Autodesk Inventor part; units mm, degrees
ref_plane "YZ Plane" through (0, 0, 0) normal (1, 0, 0) x (0, 1, 0)
ref_plane "XZ Plane" through (0, 0, 0) normal (0, 1, 0) x (-1, 0, 0)
ref_plane "XY Plane" through (0, 0, 0) normal (0, 0, 1) x (1, 0, 0)
sketch "Sketch1" plane through (0, 0, 0) normal (0, 0, 1) x (1, 0, 0)
  circle A0 centre (0, 0) radius 3.5687
  arc A1 (-6.4809, -2.9901) -> (6.4801, -2.9918) centre (0, 0) ccw
  line L0 (-20.3315, 22.225) -> (23.7148, 22.225)
  circle A2 centre (0, 44.45) radius 3.5687
  arc A3 (6.4801, 47.4418) -> (-6.4809, 47.4401) centre (0, 44.45) ccw
  circle A4 centre (0, 22.225) radius 14.8487
  circle A5 centre (0, 22.225) radius 13.5003
  line L1 (-18.1146, 22.225) -> (-6.4809, 47.4401)
  line L2 (18.1226, 22.225) -> (6.4801, 47.4418)
  line L3 (-18.1146, 22.225) -> (-6.4809, -2.9901)
  line L4 (18.1226, 22.225) -> (6.4801, -2.9918)
  point P0 (-14.3353, 14.0338)
  point P1 (14.3408, 14.0338)
  dimension "d0" = 7.1374
  dimension "d1" = 14.2748
  dimension "d2" = 44.45
extrude "Extrusion1" add sketch "Sketch1" against normal blind 1.6002
sketch "Sketch2" plane through (0, 0, 0) normal (1, 0, 0) x (0, 1, 0)
  point P0 (0, 0)
sketch "Sketch3" plane through (0, 0, 0) normal (1, 0, 0) x (0, 1, 0)
  arc A0 (35.7382, 2.1018) -> (35.0472, 13.022) centre (22.225, 6.7287) ccw
  line L0 (51.5874, 0) -> (47.4401, 0)
  line L1 (51.5874, 0) -> (34.4832, 0)
  line L2 (-2.9901, 0) -> (-7.1374, 0)
  line L3 (-7.1374, 0) -> (7.1476, 1.1293)
  line L4 (33.3323, 12.8864) -> (35.0472, 13.022)
  arc A1 (35.7382, 2.1018) -> (37.2401, 0) centre (37.2401, 1.5875) ccw
  line L5 (48.0187, -1.6002) -> (40.8813, -1.6002)
  line L6 (3.5687, -1.6002) -> (-3.5687, -1.6002)
  line L7 (22.225, -1.6002) -> (-2.9901, -1.6002)
  line L8 (47.4401, -1.6002) -> (22.225, -1.6002)
  line L9 (47.4418, -1.6002) -> (47.4401, -1.6002)
  line L10 (22.225, -1.6002) -> (47.4418, -1.6002)
  line L11 (-2.9918, -1.6002) -> (22.225, -1.6002)
  line L12 (-2.9901, -1.6002) -> (-2.9918, -1.6002)
  arc A2 (34.2371, 2.6056) -> (33.3323, 12.8864) centre (22.225, 6.7287) ccw
  line L13 (51.5874, -1.6002) -> (47.4401, -1.6002)
  line L14 (51.5874, -1.6002) -> (37.2401, -1.6002)
  arc A3 (34.2371, 2.6056) -> (34.4832, 0) centre (37.2401, 1.5748) ccw
  line L15 (22.225, -1.6002) -> (22.225, 16.2984)
  arc A4 (34.4832, 0) -> (37.2401, -1.6002) centre (37.2401, 1.5748) ccw
  line L16 (37.2401, -1.6002) -> (22.225, -1.6002)
  line L17 (34.4832, 0) -> (22.225, 0)
  point P0 (0, 0)
  point P1 (47.4418, 0)
  point P2 (-2.9918, 0)
  point P3 (31.8125, -1.6002)
  dimension "d28" = 1.5875
  dimension "d29" = 3.175
revolve "Revolution2" add sketch "Sketch3" angle 360 about axis through (0, 22.225, -1.6002) along (0, 0, 1) contours A1 L1 A3 A2 L4 A0
revolve "Revolution3" cut sketch "Sketch3" angle 360 about axis through (0, 22.225, -1.6002) along (0, 0, 1) contours A4 L8 L15 L17
sketch "Sketch4" plane through (0, 0, 0) normal (0, 0, 1) x (1, 0, 0)
  line L0 (6.4801, -2.9918) -> (18.1226, 22.225)
  line L1 (18.1226, 22.225) -> (6.4801, 47.4418)
  circle A0 centre (0, 44.45) radius 3.5687
  circle A1 centre (0, 22.225) radius 15.0151
  line L2 (0, 44.45) -> (0, 57.4596)
  line L3 (-14.2875, 44.45) -> (-14.2875, 57.4596)
  arc A2 (14.2875, 30.5316) -> (14.2875, 26.8424) centre (18.632, 28.687) ccw
  arc A3 (14.2875, 17.6076) -> (14.2875, 26.8424) centre (0, 22.225) ccw
  arc A4 (14.2875, 17.6076) -> (14.2875, 13.9184) centre (18.632, 15.763) ccw
  line L4 (14.2875, 30.5316) -> (14.2875, 57.4596)
  dimension "d33" = 14.2875
extrude "Extrusion2" cut sketch "Sketch4" against normal up to next contours A4 A1 A2 L1 L0 | A4 A1 | A1 A2
mirror "Mirror1" about plane through (0, 0, 0) normal (1, 0, 0) of "Extrusion2"
equation "\"d33\" = 0.5 * d32"
properties part number "Misc_FlangeMount_Triangle_4050"
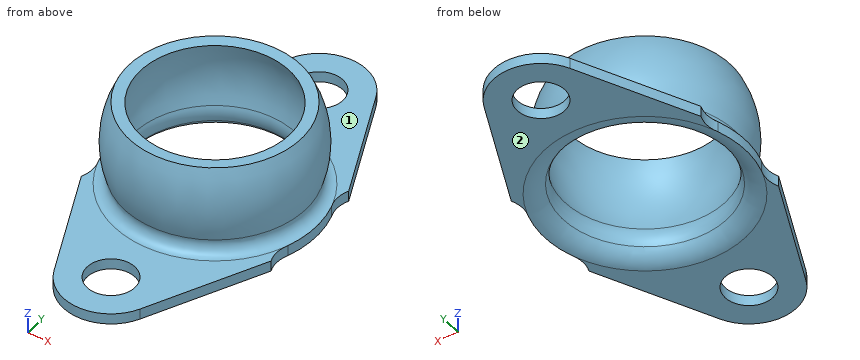
CAD build for the part. Positions are in the model's coordinates, mm. Face numbers are marked on the shaded views. A direction names the side the tool comes from. Round coordinates to 2 decimals unless told otherwise and drop trailing zeros. Order: outer loops, then holes, each group sorted by start corner. A loop starts at its lowest first (then second) coordinate and runs counter-clockwise, first axis right, second up. Notation, with made-up numbers: (83, 5) -> (98, 5) arc R20 cw to (98, 44) -> close; hole circle Ø8 at (4, 60.25). An arc over 180 degrees is marked (long way). Write item = value, one per line. Start each with the question number.
(1) Pin check, flat tips, straight feed: P1, Ø4, axis at x = -11, z = 5.5, coming from the -Y side; P2, Ø3, axis at x = -5, y = 45.5, coming from the +Z side; P3, Ø4, axis at x = 2, z = 4, coming from the +Y side. Stop position of each tip, or through.
(2) Cut at B-B, the plane x = 0. State how many separate pieces and enclosed holes the cut face has, then the cut area to 3 significant figures.
(3) Which spindle directions (+Z, -Z, +X, -X, +Y, -Y) get a long thin tool onto all of the face, cutting with end or side? Do the marked faces 1 and 2. Say none if no direction does.
(4) Probe line 1 (Y direction, x = 0, z = -0.9); line 2 (Y direction, x = 0, z = -1.15); line 3 (Z direction, x = -2.5, y = 3). List the from-to ranges inside material, lowest first. Write a range as [from, to].
(5) Cut at A-A, the plane y = 0. List the corners of the cut face in (x, z).
(6) Cut at C-C, the plane y = 46. List the corners of the cut face in (x, z).
Model answer:
q1.P1 = 11.19
q1.P2 = 0
q1.P3 = 36.44
q2.separate_pieces = 4
q2.enclosed_holes = 0
q2.area = 72.1 mm2
q3.face_1 = +Z, +Y
q3.face_2 = -Z, +X, -X, +Y, -Y
q4.line_1 = [-7.14, -3.57], [3.57, 9.2], [35.25, 40.88], [48.02, 51.59]
q4.line_2 = [-7.14, -3.57], [3.57, 8.84], [35.61, 40.88], [48.02, 51.59]
q4.line_3 = [-1.6, 0]
q5.outline = (-7.86, -1.6) -> (-3.57, -1.6) -> (-3.57, 0) -> (-7.86, 0) -> close; (3.57, -1.6) -> (7.86, -1.6) -> (7.86, 0) -> (3.57, 0) -> close
q6.outline = (-7.15, -1.6) -> (-3.21, -1.6) -> (-3.21, 0) -> (-7.15, 0) -> close; (3.21, -1.6) -> (7.15, -1.6) -> (7.15, 0) -> (3.21, 0) -> close
